from build123d import *

# Parameters (mm, degrees)
BOSS_EXTRUDE1_DEPTH = 8.128
SKETCH2_W           = 7.62
SKETCH2_H           = 0.635
CUT_EXTRUDE1_DEPTH  = 6.35


with BuildPart() as part:
    # Sketch1 → Boss-Extrude1 (new body)
    with BuildSketch(Plane.XY):
        Polygon((-4.699, 10.16), (-4.699, 9.652), (0, 9.652), (0, 0), (1.016, 0), (1.016, 9.144), (12.192, 9.144), (12.192, 0), (13.208, 0), (13.208, 9.652), (17.907, 9.652), (17.907, 10.16), (12.192, 10.16), (12.192, 9.652), (1.016, 9.652), (1.016, 10.16), align=None)
    extrude(amount=BOSS_EXTRUDE1_DEPTH)

    # Sketch2 → Cut-Extrude1 (cut)
    with BuildSketch(Plane(origin=(0, 10.16, 0), x_dir=(1, 0, 0), z_dir=(0, 1, 0))):
        with Locations((0.889, -2.159)):
            Rectangle(SKETCH2_W, SKETCH2_H)
        with Locations((0.889, -4.064)):
            Rectangle(SKETCH2_W, SKETCH2_H)
        with Locations((0.889, -5.969)):
            Rectangle(SKETCH2_W, SKETCH2_H)
        with Locations((12.319, -2.159)):
            Rectangle(SKETCH2_W, SKETCH2_H)
        with Locations((12.319, -4.064)):
            Rectangle(SKETCH2_W, SKETCH2_H)
        with Locations((12.319, -5.969)):
            Rectangle(SKETCH2_W, SKETCH2_H)
    extrude(amount=-CUT_EXTRUDE1_DEPTH, mode=Mode.SUBTRACT)


solid = part.part
Design review of the part built by this model. Coordinates are the model's own, in mm. A direction names the side the tool comes from. Round coordinates to 2 decimals unless told otherwise and drop trailing zeros. Loops run counter-clockwise (first coordinate to the right, second up) from the corner with the lowest first, then second, coordinate; pieces in that order, holes last. Notation, with made-up numbers: M 64,20.5 L 81,20.5 A24 cw 81,34.5 Z; hole C -32,-22.5 d3. An arc over 180 degrees is marked long. Answer as a JSON object with one key per item and string values.
Item 1: Machinability: for faces 1 (the flat face through (17, 9.652, 4)), 2 (the flat face through (7, 9.652, 4)), 3 (the flat face through (0.6, 7.9, 1.842)), 4 (the flat face through (12.192, 3.6, 4)), which of the approach directions +Z, -Z, +X, -X, +Y, -Y give a long, thin tool a straight path to every point of the face, cutting with its end or side? Answer none if there is none.
Answer sheet:
{"face 1": "+Z, -Z, +X, -Y", "face 2": "+Z, -Z, +Y", "face 3": "+Y", "face 4": "+Z, -Z, -Y"}
Item 2: Wall thickness on L1, parallel to Z at x = 12.25, y = 6.5; L2, parallel to X at y = 6.25, z = 1; L3, parallel to X at y = 9.75, z = 2.75: over which ranges is each line inside the solid? List them lowest first. Write a range as from..to.
Answer sheet:
{"L1": "z = 0..1.84, 2.48..3.75, 4.38..5.65, 6.29..8.13", "L2": "x = 0..1.02, 12.19..13.21", "L3": "x = -4.7..1.02, 12.19..17.91"}
Item 3: We need section B-B on x = 14.25. Give the boundary of the cut face in (y, z).
Answer sheet:
{"outline": "M 9.65,0 L 10.16,0 L 10.16,1.84 L 9.65,1.84 Z; M 9.65,2.48 L 10.16,2.48 L 10.16,3.75 L 9.65,3.75 Z; M 9.65,4.38 L 10.16,4.38 L 10.16,5.65 L 9.65,5.65 Z; M 9.65,6.29 L 10.16,6.29 L 10.16,8.13 L 9.65,8.13 Z"}
Item 4: The part is to be moulded in two halves that separate along X. For faces 5 (the flat face through (0, 5, 5)), 6 (the flat face through (0.6, 7.9, 5.652)), 7 (the flat face through (0.5, 0, 4)), say which applies: pulls with the +X half, pulls with the -X half, needs draft (parallel to the pull), parting line crosses it, or undercut.
Answer sheet:
{"face 5": "pulls with the -X half", "face 6": "undercut", "face 7": "needs draft"}
Item 5: We need section A-A on y = 2. Give the boundary of the cut face in (x, z), and give its area (3 significant figures).
Answer sheet:
{"outline": "M 0,0 L 1.02,0 L 1.02,8.13 L 0,8.13 Z; M 12.19,0 L 13.21,0 L 13.21,8.13 L 12.19,8.13 Z", "area": "16.5 mm^2"}
Item 6: Clearance check with a flat-ended pin moving along its axis: P1, Ø2, axis at x = 2.5, z = 4, coming from the -Y side. State where the tip first meets the part, or that it passes through.
Answer sheet:
{"P1": "stops at y = 9.14"}
Item 7: We need section C-C on y = 8.5. State how many separate pieces and enclosed holes the cut face has, and give its area (3 significant figures).
Answer sheet:
{"separate pieces": "8", "enclosed holes": "0", "area": "12.6 mm^2"}
Item 8: We need section D-D on z = 6. Give the boundary of the cut face in (x, y), and give its area (3 significant figures).
Answer sheet:
{"outline": "M -4.7,9.65 L -2.92,9.65 L -2.92,10.16 L -4.7,10.16 Z; M 0,0 L 1.02,0 L 1.02,3.81 L 0,3.81 Z; M 4.7,9.14 L 8.51,9.14 L 8.51,9.65 L 4.7,9.65 Z; M 12.19,0 L 13.21,0 L 13.21,3.81 L 12.19,3.81 Z; M 16.13,9.65 L 17.91,9.65 L 17.91,10.16 L 16.13,10.16 Z", "area": "11.5 mm^2"}
